Build history of the part. All positions in model axes, mm. Round coordinates to 2 decimals unless told otherwise and drop trailing zeros. Write each loop counter-clockwise with the first axis right and the second up, starting at its lowest first coordinate (ties: lowest second). Pieces come first, ordered by that corner, then holes.
1) Saw through at A-A (z = 0). Write the cut outline in (x, y), plus the area to 3 significant figures.
2) Wall check: probe 1 along X at (y, z) = (-0.5, 13); probe 2 along X at (y, z) = (-25, -2); probe 3 along Y at (x, z) = (9.5, -13.5). Give the ranges that are in metal, low to high.
3) Flat gauge pins, fed straight in: pin 1 (4 mm diameter, centred on x = -19, z = 6.5, fed in from +Y); pin 2 (1 mm diameter, centred on y = -21.5, z = -9, fed in from -X); pin 3 (1 mm diameter, centred on x = -20.5, z = 4.5, fed in from +Y). Where does each tip first touch, or does it go through?
from build123d import *

# Parameters (mm, degrees)
CYLINDER038_R     = 30
CYLINDER038_DEPTH = 32
CHAMFER010_SIZE   = 2
CHAMFER011_SIZE   = 2


with BuildPart() as part:
    # Cylinder038 → Cylinder038 (join)
    with BuildSketch(Plane.XY.offset(-16)):
        Circle(CYLINDER038_R)
    extrude(amount=CYLINDER038_DEPTH)

    # Chamfer010
    chamfer010_edges = [part.edges().sort_by_distance(p)[0] for p in [
        (-30, 0, 16),
    ]]
    chamfer(chamfer010_edges, length=CHAMFER010_SIZE)

    # Chamfer011
    chamfer011_edges = [part.edges().sort_by_distance(p)[0] for p in [
        (-30, 0, -16),
    ]]
    chamfer(chamfer011_edges, length=CHAMFER011_SIZE)


solid = part.part
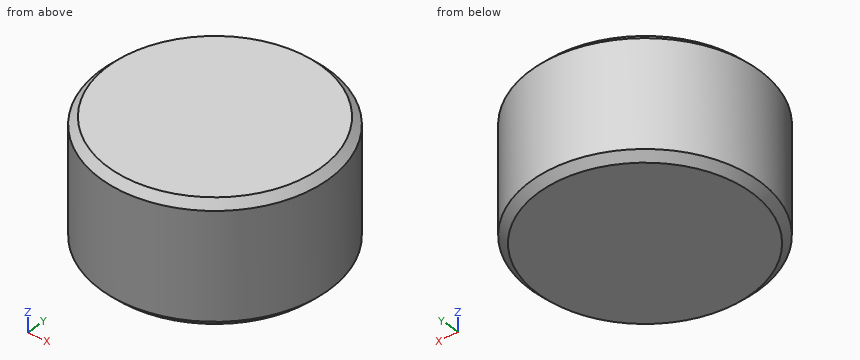
Evaluation:
1. outline: circle Ø60 at (0, 0)
1. area: 2,830 mm2
2. probe 1: x = -30 to 30
2. probe 2: x = -16.58 to 16.58
2. probe 3: y = -28.46 to 28.46
3. pin 1: stops at y = 24.72
3. pin 2: stops at x = -21.42
3. pin 3: stops at y = 22.36
